```python
from build123d import *

# Parameters (mm, degrees)
BOSS_EXTRUDE1_DEPTH = 10
DRAFT1_ANGLE        = 45
BOSS_EXTRUDE2_DEPTH = 30
SKETCH6_W           = 50
SKETCH6_H           = 17.7
BOSS_EXTRUDE3_DEPTH = 50
SKETCH7_W           = 50
SKETCH7_H           = 7.7
CUT_EXTRUDE4_DEPTH  = 20
CHAMFER1_SIZE       = 10


with BuildPart() as part:
    # Sketch2 → Boss-Extrude1 (new body)
    with BuildSketch(Plane(origin=(0, 0, 0), x_dir=(1, 0, 0), z_dir=(0, 1, 0))):
        Polygon((-90, 5), (90, 5), (120, -55), (115.527864045, -57.236067977), (88.291796068, -2.763932023), (-88.291796068, -2.763932023), (-115.527864045, -57.236067977), (-120, -55), align=None)
    extrude(amount=BOSS_EXTRUDE1_DEPTH)

    # Draft1
    draft1_faces = [part.faces().sort_by_distance(p)[0] for p in [
        (101.909830056, 5, 30),
        (0, 5, 2.763932023),
        (-101.909830056, 5, 30),
    ]]
    draft(draft1_faces, Plane.ZX.offset(10), DRAFT1_ANGLE)

    # Sketch5 → Boss-Extrude2 (add)
    with BuildSketch(Plane(origin=(0, 10, 0), x_dir=(1, 0, 0), z_dir=(0, 1, 0))):
        Polygon((-120, -55), (-90, 5), (90, 5), (120, -55), (115.527864045, -57.236067977), (88.291796068, -2.763932023), (-88.291796068, -2.763932023), (-115.527864045, -57.236067977), align=None)
    extrude(amount=BOSS_EXTRUDE2_DEPTH)

    # Sketch6 → Boss-Extrude3 (add)
    with BuildSketch(Plane(origin=(0, 0, -5), x_dir=(-1, 0, 0), z_dir=(0, 0, -1))):
        with Locations((0, 14.45)):
            Rectangle(SKETCH6_W, SKETCH6_H)
    extrude(amount=BOSS_EXTRUDE3_DEPTH)

    # Sketch7 → Cut-Extrude4 (cut)
    with BuildSketch(Plane(origin=(0, 0, -55), x_dir=(-1, 0, 0), z_dir=(0, 0, -1))):
        with Locations((0, 14.45)):
            Rectangle(SKETCH7_W, SKETCH7_H)
    extrude(amount=-CUT_EXTRUDE4_DEPTH, mode=Mode.SUBTRACT)

    # Chamfer1
    # the kernel refuses this chamfer: 10 mm, written as the material it takes off along each edge
    with BuildSketch(Plane(origin=(78.499084045, 0, -28.001831911), x_dir=(-0.8940890232049223, -0.027495876610586386, 0.44704451160246145), z_dir=(0.44721359549995815, 0, 0.8944271909999159))) as chamfer1_piece_1:
        Polygon((CHAMFER1_SIZE * 0.999621916911, -CHAMFER1_SIZE * 0.0274958766106), (-CHAMFER1_SIZE * 0.0274958766106, -CHAMFER1_SIZE * 0.999621916911), (0, 0), align=None)
    extrude(amount=118.515699084, mode=Mode.SUBTRACT)
    with BuildSketch(Plane(origin=(-115.71682988, 0, -5), x_dir=(0, 0.9996219169112968, -0.027495876610586403), z_dir=(1, 0, 0))) as chamfer1_piece_2_section:
        Polygon((CHAMFER1_SIZE * 0.999621916911, CHAMFER1_SIZE * 0.0274958766106), (-CHAMFER1_SIZE * 0.0274958766106, CHAMFER1_SIZE * 0.999621916911), (0, 0), align=None)
    chamfer1_piece_2 = extrude(amount=231.433659759, mode=Mode.PRIVATE)
    chamfer1_piece_2 = split(chamfer1_piece_2, bisect_by=Plane(origin=(-70.35841494, 5.6, -3.753576162), z_dir=(0, 1, 0)), keep=Keep.TOP, mode=Mode.PRIVATE)
    chamfer1_piece_2 = split(chamfer1_piece_2, bisect_by=Plane(origin=(-25, 7.219915687, -3.753576162), z_dir=(-1, 0, 0)), keep=Keep.TOP, mode=Mode.PRIVATE)
    add(chamfer1_piece_2, mode=Mode.SUBTRACT)
    with BuildSketch(Plane(origin=(-115.71682988, 0, -5), x_dir=(0, 0.9996219169112968, -0.027495876610586403), z_dir=(1, 0, 0))) as chamfer1_piece_3_section:
        Polygon((CHAMFER1_SIZE * 0.999621916911, CHAMFER1_SIZE * 0.0274958766106), (-CHAMFER1_SIZE * 0.0274958766106, CHAMFER1_SIZE * 0.999621916911), (0, 0), align=None)
    chamfer1_piece_3 = extrude(amount=231.433659759, mode=Mode.PRIVATE)
    chamfer1_piece_3 = split(chamfer1_piece_3, bisect_by=Plane(origin=(-70.35841494, 5.6, -1.178972158), z_dir=(0, -1, 0)), keep=Keep.TOP, mode=Mode.PRIVATE)
    chamfer1_piece_3 = split(chamfer1_piece_3, bisect_by=Plane(origin=(-25, 2.297915816, -1.178972158), z_dir=(-1, 0, 0)), keep=Keep.TOP, mode=Mode.PRIVATE)
    add(chamfer1_piece_3, mode=Mode.SUBTRACT)
    with BuildSketch(Plane(origin=(-115.71682988, 0, -5), x_dir=(0, 0.9996219169112968, -0.027495876610586403), z_dir=(1, 0, 0))) as chamfer1_piece_4_section:
        Polygon((CHAMFER1_SIZE * 0.999621916911, CHAMFER1_SIZE * 0.0274958766106), (-CHAMFER1_SIZE * 0.0274958766106, CHAMFER1_SIZE * 0.999621916911), (0, 0), align=None)
    chamfer1_piece_4 = extrude(amount=231.433659759, mode=Mode.PRIVATE)
    chamfer1_piece_4 = split(chamfer1_piece_4, bisect_by=Plane(origin=(0, 5.6, -1.178972158), z_dir=(0, -1, 0)), keep=Keep.TOP, mode=Mode.PRIVATE)
    chamfer1_piece_4 = split(chamfer1_piece_4, bisect_by=Plane(origin=(-25, 2.297915816, -1.178972158), z_dir=(1, 0, 0)), keep=Keep.TOP, mode=Mode.PRIVATE)
    chamfer1_piece_4 = split(chamfer1_piece_4, bisect_by=Plane(origin=(25, 2.297915816, -1.178972158), z_dir=(-1, 0, 0)), keep=Keep.TOP, mode=Mode.PRIVATE)
    add(chamfer1_piece_4, mode=Mode.SUBTRACT)
    with BuildSketch(Plane(origin=(-115.71682988, 0, -5), x_dir=(0, 0.9996219169112968, -0.027495876610586403), z_dir=(1, 0, 0))) as chamfer1_piece_5_section:
        Polygon((CHAMFER1_SIZE * 0.999621916911, CHAMFER1_SIZE * 0.0274958766106), (-CHAMFER1_SIZE * 0.0274958766106, CHAMFER1_SIZE * 0.999621916911), (0, 0), align=None)
    chamfer1_piece_5 = extrude(amount=231.433659759, mode=Mode.PRIVATE)
    chamfer1_piece_5 = split(chamfer1_piece_5, bisect_by=Plane(origin=(70.35841494, 5.6, -3.753576162), z_dir=(0, 1, 0)), keep=Keep.TOP, mode=Mode.PRIVATE)
    chamfer1_piece_5 = split(chamfer1_piece_5, bisect_by=Plane(origin=(25, 7.219915687, -3.753576162), z_dir=(1, 0, 0)), keep=Keep.TOP, mode=Mode.PRIVATE)
    add(chamfer1_piece_5, mode=Mode.SUBTRACT)
    with BuildSketch(Plane(origin=(-115.71682988, 0, -5), x_dir=(0, 0.9996219169112968, -0.027495876610586403), z_dir=(1, 0, 0))) as chamfer1_piece_6_section:
        Polygon((CHAMFER1_SIZE * 0.999621916911, CHAMFER1_SIZE * 0.0274958766106), (-CHAMFER1_SIZE * 0.0274958766106, CHAMFER1_SIZE * 0.999621916911), (0, 0), align=None)
    chamfer1_piece_6 = extrude(amount=231.433659759, mode=Mode.PRIVATE)
    chamfer1_piece_6 = split(chamfer1_piece_6, bisect_by=Plane(origin=(70.35841494, 5.6, -1.178972158), z_dir=(0, -1, 0)), keep=Keep.TOP, mode=Mode.PRIVATE)
    chamfer1_piece_6 = split(chamfer1_piece_6, bisect_by=Plane(origin=(25, 2.297915816, -1.178972158), z_dir=(1, 0, 0)), keep=Keep.TOP, mode=Mode.PRIVATE)
    add(chamfer1_piece_6, mode=Mode.SUBTRACT)
    with BuildSketch(Plane(origin=(-131.500915955, 0, 78.001831911), x_dir=(-0.02459305968088589, 0.9996219169112968, -0.012296529840442941), z_dir=(0.447213595499958, 0, -0.894427190999916))) as chamfer1_piece_7:
        Polygon((CHAMFER1_SIZE * 0.999621916911, CHAMFER1_SIZE * 0.0274958766106), (-CHAMFER1_SIZE * 0.0274958766106, CHAMFER1_SIZE * 0.999621916911), (0, 0), align=None)
    extrude(amount=118.515699084, mode=Mode.SUBTRACT)


solid = part.part
```
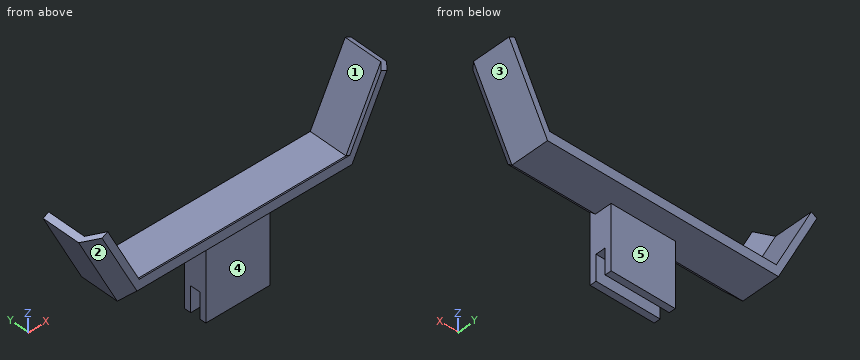
Part model, mm, in its own coordinate system. Face numbers are marked on the shaded views. A direction names the side the tool comes from. Round coordinates to 2 decimals unless told otherwise and drop trailing zeros. Loops run counter-clockwise (first coordinate to the right, second up) from the corner with the lowest first, then second, coordinate; pieces in that order, holes last.
1. Slice it at B-B (z = 49). Give the cut face in (x, y), and give its area (3 significant figures).
Solutions:
outline: (-117, 10) - (-105.82, 0) - (-100.23, 0) - (-111.41, 10) - (-111.41, 40) - (-117, 40) - close; (100.23, 0) - (105.82, 0) - (117, 10) - (117, 40) - (111.41, 40) - (111.41, 10) - close
area: 447 mm2
2. Flat gauge pins, fed straight in: pin 1 (1 mm diameter, centred on x = 1.5, y = 34, fed in from -Z); pin 2 (22 mm diameter, centred on x = -4, z = -43, fed in from -Y); pin 3 (2.5 mm diameter, centred on x = 5.5, y = 15, fed in from -Z); pin 4 (10 mm diameter, centred on x = 15, z = 21, fed in from -Y). Where does each tip first touch, or does it go through?
Solutions:
pin 1: stops at z = -5
pin 2: stops at y = 5.6
pin 3: stops at z = -35
pin 4: passes through
3. Slice it at D-D (z = -38). Give the cut face in (x, y).
Solutions:
outline: (-25, 5.6) - (25, 5.6) - (25, 10.6) - (-25, 10.6) - close; (-25, 18.3) - (25, 18.3) - (25, 23.3) - (-25, 23.3) - close
4. Slice it at C-C (x = -4). Give the cut face in (y, z), and give its area (3 significant figures).
Solutions:
outline: (0, 5) - (5.6, -0.6) - (5.6, -55) - (10.6, -55) - (10.6, -35) - (18.3, -35) - (18.3, -55) - (23.3, -55) - (23.3, -5) - (40, -5) - (40, 2.76) - (10, 2.76) - (0, 12.76) - close
area: 1,050 mm2
5. 3-axis set-ups, long thin cutter, end or side, ignore diameter. For the marked faces 1, 2, 3, 4 and 5: which of +Z, -Z, +X, -X, +Y, -Y reach the whole face in a straight line?
Solutions:
face 1: +Z, +Y
face 2: -Z, -X, -Y
face 3: -Z, +X, +Y, -Y
face 4: -Z, +X, -X, -Y
face 5: -Z, +X, -X, +Y
6. Slice it at A-A (y = 25.5). Give the cut face in (x, z), and give its area (3 significant figures).
Solutions:
outline: (-120, 55) - (-90, -5) - (90, -5) - (120, 55) - (115.53, 57.24) - (88.29, 2.76) - (-88.29, 2.76) - (-115.53, 57.24) - close
area: 2,020 mm2
7. Drill centre lines: line 1 along X through (y, z) = (30.5, 31); line 2 along Z through (x, y) = (-41.5, 36); line 3 along Z through (x, y) = (15, 12). Where is each one in solid material? Low to high.
Solutions:
line 1: x = -108 to -102.41, 102.41 to 108
line 2: z = -5 to 2.76
line 3: z = -35 to 2.76
